```python
from build123d import *

# Parameters (mm, degrees)
F1_DEPTH      = 2
F2_R          = 2.0000003278
F2_R_2        = 1
F3_DEPTH      = 4.325
F3_DEPTH_BACK = 4.325
F4_W          = 0.9
F4_H          = 2.5
F5_DEPTH      = 3.0010606999


with BuildPart() as f1:
    # F0 (on Top) → F1 (new body)
    with BuildSketch(Plane.XY):
        Polygon((-10.25, 25.5), (0, 25.5), (10.25, 25.5), (10.25, 28), (0, 28), (-10.25, 28), align=None)
        Polygon((-17, 45), (-10.25, 28), (0, 28), (10.25, 28), (17, 45), (0, 45), align=None)
        Polygon((-17, 57), (-17, 45), (0, 45), (17, 45), (17, 57), (0, 57), align=None)
    extrude(amount=F1_DEPTH)

    # F2 (on Right) → F3 (join, two sides)
    with BuildSketch(Plane.YZ) as f3_sk:
        with Locations((23.7735025585, 0.9999396279)):
            Circle(F2_R)
        with Locations((23.7735025585, 0.9999396279)):
            Circle(F2_R_2, mode=Mode.SUBTRACT)
    extrude(amount=-F3_DEPTH)
    extrude(f3_sk.sketch, amount=F3_DEPTH_BACK)

    # F4 (on face) → F5 (cut, through all)
    with BuildSketch(Plane.XY.offset(2)):
        with Locations((4.775, 26.75)):
            Rectangle(F4_W, F4_H)
        with Locations((-4.775, 26.75)):
            Rectangle(F4_W, F4_H)
    extrude(amount=-F5_DEPTH, mode=Mode.SUBTRACT)


solid = f1.part
```
Input: part model. Units: mm. Frame: model coordinates. A direction names the side the tool comes from. Give positions to 0.01 mm unless a question says otherwise; leave off trailing zeros. Loops run counter-clockwise (first coordinate to the right, second up) from the corner with the lowest first, then second, coordinate; pieces in that order, holes last. Notation, with made-up numbers: M 25.25,45.25 L 78.25,45.25 A21 ccw 78.25,67.25 Z; hole C 6,56 d6. An arc over 180 degrees is marked long. Answer as CSV lines item,"result". Start each with the question number.
1. Section C-C on x = 9. Return loops of the section in (y, z).
2. Pull-direction query (X, two-part tool) for faces 1 (the face through (8, 25.5, 1)), 2 (the face through (13.578, 36.381, 0.986)), 3 (the face through (-4.325, 25, 1)); classes: released by +X, released by -X, zero draft, split by the parting line, or undercut.
3. Reachability of faces 4 (the face through (-5, 28, 1)), 5 (the face through (-8, 25.5, 1)), 6 (the face through (10.25, 27, 1)), 7 (the face through (0, 41, 2)) from +Z, -Z, +X, -X, +Y, -Y: full face, straight path, thin tool, end or side. Return the list, or none.
4. Line query: L1, parallel to Y at x = 10, z = 1; L2, parallel to Y at x = 0.5, z = 1.1; L3, parallel to Z at x = -4, y = 34. Output: solid intervals per line, ascending.
5. Section A-A on y = 55. Return loops of the section in (x, z).
6. Section B-B on x = 3. Return loops of the section in (y, z).
7. Pin query (flat end, axial travel): P1, Ø1.5, axis at x = 4, y = 26.5, coming from the +Z side; P2, Ø5, axis at x = 2.5, y = 26.5, coming from the +Z side; P3, Ø1, axis at y = 26.5, z = 1, coming from the +X side. Return the tip coordinate at first contact, or that it passes through.
Computed values:
1,outline,"M 25.5,0 L 57,0 L 57,2 L 25.5,2 Z"
2,face 1,"zero draft"
2,face 2,"released by +X"
2,face 3,"undercut"
3,face 4,"+Z, -Z, -Y"
3,face 5,"+Z, -Z, -X, -Y"
3,face 6,"+Z, -Z, +X, -Y"
3,face 7,"+Z, +X, -X, +Y"
4,L1,"y = 25.5 to 57"
4,L2,"y = 21.78 to 22.78, 24.77 to 57"
4,L3,"z = 0 to 2"
5,outline,"M -17,0 L 17,0 L 17,2 L -17,2 Z"
6,outline,"M 25.51,0 L 57,0 L 57,2 L 25.51,2 A2 ccw long Z; hole C 23.77,1 d2"
7,P1,"stops at z = 2"
7,P2,"stops at z = 2.99"
7,P3,"stops at x = 10.25"
